Design review of the part shown in the three views and the two pictorial views. Dimensions are in mm from the part's minimum x, y and z. A direction names the side the tool comes from. Coordinates: 2 decimals unless noted, no trailing zeros. Loops run counter-clockwise (first coordinate to the right, second up) from the corner with the lowest first, then second, coordinate; pieces in that order, holes last. Notation, with made-up numbers: (-35, 82.5) - (-15, 82.5) arc R9 cw to (-15, 91.5) - close; hole circle Ø10 at (2, 73.25). An arc over 180 degrees is marked (long way). One line per question, with ' | ' between items.
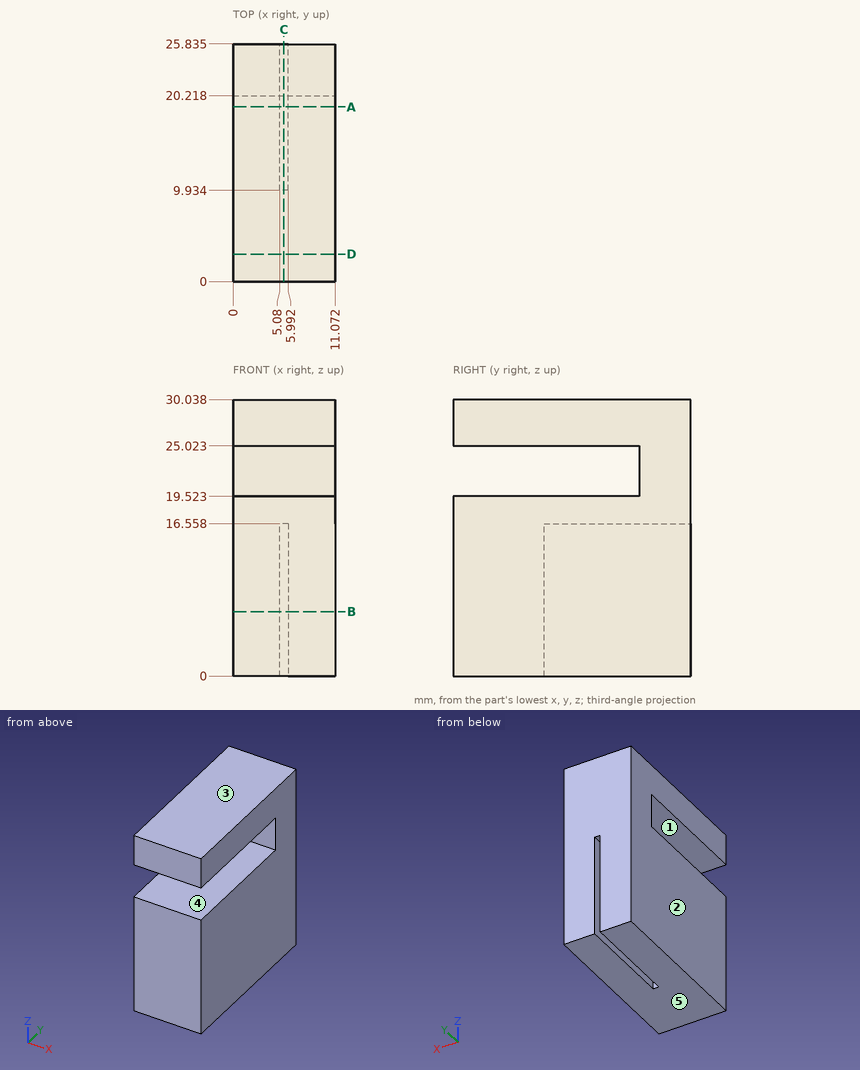
Q1. Draft analysis for pull direction Z (two halves, no side actions). For the marked faces 1, 2 and 3, state which applies: +Z half, -Z half, draft (parallel to the pull), parting line (faces both ways), or undercut.
Returned:
face 1: undercut | face 2: draft | face 3: +Z half
Q2. Take a section at C-C (x = 5.5). Give the boundary of the cut face in (y, z) (1 decimal).
Returned:
outline: (0, 0) - (9.9, 0) - (9.9, 16.6) - (25.8, 16.6) - (25.8, 30) - (0, 30) - (0, 25) - (20.2, 25) - (20.2, 19.5) - (0, 19.5) - close
Q3. For pin 1 (1.7 mm diameter, centred on x = 4, z = 21, fed in from -Y); pin 2 (0.7 mm diameter, centred on x = 5.5, z = 4.5, fed in from +Y), all flat-tipped, find the tip position at first contact; note any pin that passes through.
Returned:
pin 1: stops at y = 20.22 | pin 2: stops at y = 9.93
Q4. To check wall thickness, follow line 1 along Z through (x, y) = (3.25, 18.25); line 2 along X through (y, z) = (13.25, 14.5); line 3 along Y through (x, z) = (6.5, 21.5) (1 decimal). State the ranges of each line that lie inside material, in increasing order.
Returned:
line 1: z = 0 to 19.52, 25.02 to 30.04 | line 2: x = 0 to 5.08, 5.99 to 11.07 | line 3: y = 20.2 to 25.8
Q5. Take a section at B-B (z = 7). Give the boundary of the cut face in (x, y) (1 decimal).
Returned:
outline: (0, 0) - (11.1, 0) - (11.1, 25.8) - (6, 25.8) - (6, 9.9) - (5.1, 9.9) - (5.1, 25.8) - (0, 25.8) - close
Q6. Tool access review of the marked faces 4 and 5: name each direction out of +Z, -Z, +X, -X, +Y, -Y from which nothing blocks a thin tool from reaching the whole face with its end or side.
Returned:
face 4: +X, -X, -Y | face 5: -Z, +X, -X, +Y, -Y
Q7. Take a section at D-D (y = 3). Give the boundary of the cut face in (x, z), plus the area to 3 significant figures.
Returned:
outline: (0, 0) - (11.07, 0) - (11.07, 19.52) - (0, 19.52) - close; (0, 25.02) - (11.07, 25.02) - (11.07, 30.04) - (0, 30.04) - close | area: 272 mm²
Q8. Take a section at A-A (y = 19). Give the boundary of the cut face in (x, z).
Returned:
outline: (0, 0) - (5.08, 0) - (5.08, 16.56) - (5.99, 16.56) - (5.99, 0) - (11.07, 0) - (11.07, 19.52) - (0, 19.52) - close; (0, 25.02) - (11.07, 25.02) - (11.07, 30.04) - (0, 30.04) - close
